Source: three-view drawing plus pictorial views. Frame: mm from the lowest corner of the part. A direction names the side the tool comes from. Coordinates: 2 decimals unless noted, no trailing zeros. Write each loop counter-clockwise with the first axis right and the second up, starting at its lowest first coordinate (ties: lowest second). Pieces come first, ordered by that corner, then holes.
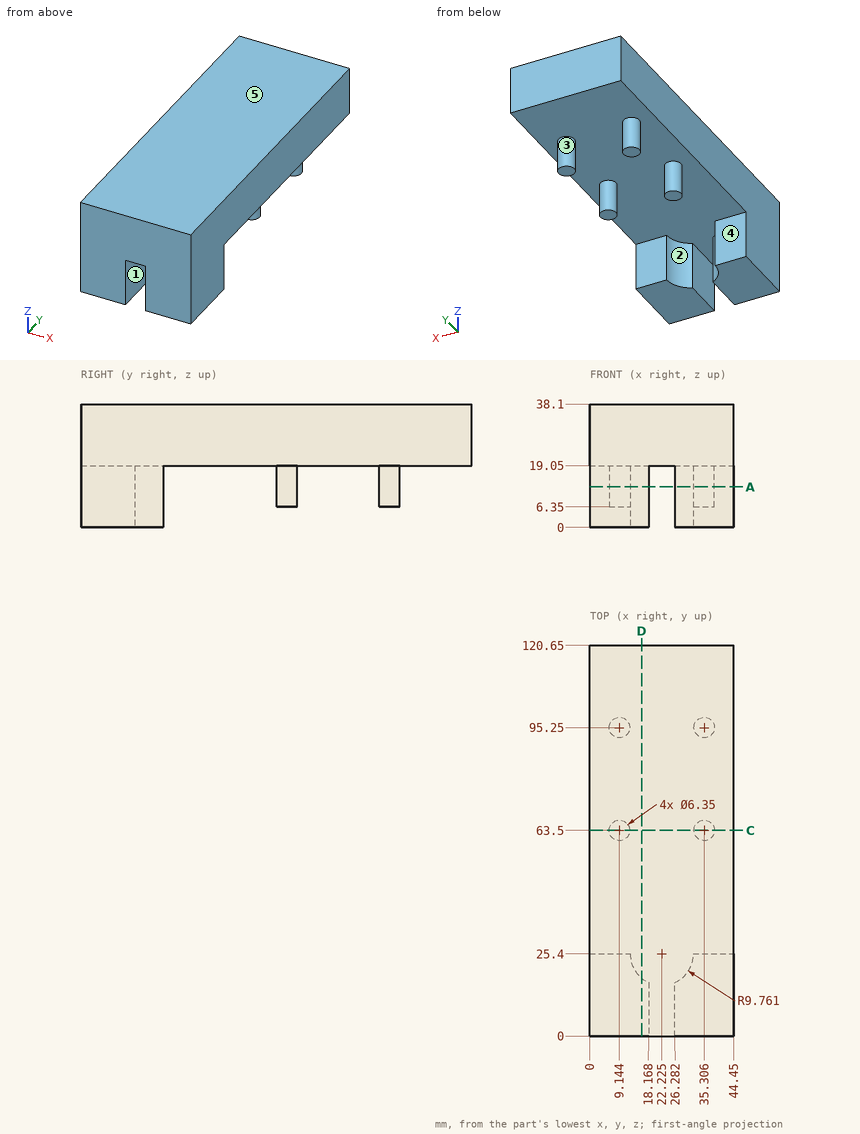
Item 1: Section query C-C, the plane y = 63.5. Return loops of the section in (x, z).
Item 2: Material intervals for line 1 (Y direction, x = 34.5, z = 8); line 2 (Y direction, x = 34, z = 11); line 3 (Z direction, x = 22, y = 68), sorted ascending.
Item 3: Access query for the marked faces 1, 2, 3, 4 and 5. Directions: +Z, -Z, +X, -X, +Y, -Y. A direction counts if a zero-diameter tool reaches every point of the face in a straight line with its end or side. Return the directions, or none.
Item 4: Pin query (flat end, axial travel): pin 1 Ø6 at (x, y) = (31.5, 62.5) entering from -Z; pin 2 Ø3 at (x, y) = (40, 49.5) entering from -Z; pin 3 Ø10 at (x, z) = (9.5, 14) entering from +Y (3 decimals). Return the tip coordinate at first contact, or that it passes through.
Item 5: Section query D-D, the plane x = 16. Return loops of the section in (y, z).
Item 6: Section query A-A, the plane z = 12.5. State how many separate pieces and enclosed holes the cut face has, then the cut area to 3 significant figures.
The answers:
1. outline: (0, 19.05) - (5.97, 19.05) - (5.97, 6.35) - (12.32, 6.35) - (12.32, 19.05) - (32.13, 19.05) - (32.13, 6.35) - (38.48, 6.35) - (38.48, 19.05) - (44.45, 19.05) - (44.45, 38.1) - (0, 38.1) - close
2. line 1: y = 0 to 25.4, 60.43 to 66.57, 92.18 to 98.32
2. line 2: y = 0 to 25.4, 60.61 to 66.39, 92.36 to 98.14
2. line 3: z = 19.05 to 38.1
3. face 1: -Z, +Y, -Y
3. face 2: -Z, +Y
3. face 3: -Z
3. face 4: -Z, +X, -X
3. face 5: +Z, +X, -X, +Y, -Y
4. pin 1: stops at z = 6.35
4. pin 2: stops at z = 19.05
4. pin 3: stops at y = 98.425
5. outline: (0, 0) - (17.88, 0) - (17.88, 19.05) - (120.65, 19.05) - (120.65, 38.1) - (0, 38.1) - close
6. separate pieces: 6
6. enclosed holes: 0
6. area: 977 mm2
